The model under review builds one solid part; all positions refer to its coordinate system, in mm. Round coordinates to 2 decimals unless told otherwise and drop trailing zeros. Write each loop counter-clockwise with the first axis right and the second up, starting at its lowest first coordinate (ties: lowest second). Pieces come first, ordered by that corner, then holes. Notation, with made-up numbers: M 16.25,26.25 L 52.25,26.25 A36 ccw 52.25,65.25 Z; hole C 53.25,88.25 d1. An arc over 180 degrees is marked long. Write item = value, one per line. Start each with the question number.
Item 1: Take a section at A-A, the plane z = 45.4. Give the boundary of the cut face in (x, y).
Item 2: The part is to be moulded in two halves that separate along Z. For faces 1 (the flat face through (-1, 0, 24)), 2 (the cylindrical face through (8.689, 14.506, 36.984)), 3 (the cylindrical face through (8.69, 14.51, -31.26)), say which applies: +Z half, -Z half, draft (parallel to the pull), parting line (faces both ways), or undercut.
Item 3: For pin 1 Ø12 at (y, z) = (21, 13.5) entering from -X; pin 2 Ø1 at (x, y) = (-3.5, 17.5) entering from +Z; pin 3 Ø6 at (x, y) = (17.5, 30) entering from +Z, all flat-tipped, find the tip position at first contact; note any pin that passes through.
Item 4: Take a section at B-B, the plane y = 33. Give the number of separate pieces and of enclosed holes in the cut face, plus the area to 3 significant figures.
Item 5: To check wall thickness, follow line 1 along Z through (x, y) = (-0.5, 21); line 2 along X through (y, z) = (19.5, 28); line 3 along X through (y, z) = (15.5, 21.5). State the ranges of each line that lie inside material, in increasing order.
from build123d import *

# Parameters (mm, degrees)
SKETCH1_R                 = 50.8
SKETCH1_R_2               = 23.5
BOSS_EXTRUDE1_DEPTH       = 7.7
SKETCH3_R                 = 50.8
SKETCH3_R_2               = 30
BOSS_EXTRUDE2_DEPTH       = 9.7625
SKETCH4_R                 = 50.8
SKETCH4_R_2               = 40
BOSS_EXTRUDE3_DEPTH       = 19.05
SKETCH5_R                 = 3
CUT_EXTRUDE1_DEPTH        = 4.7625
CHAMFER1_SIZE             = 1.2
CUT_EXTRUDE4_DEPTH        = 81.58810493
M4X0_7_TAPPED_HOLE1_D     = 3.3
M4X0_7_TAPPED_HOLE1_DEPTH = 36.5135


with BuildPart() as part:
    # Sketch1 → Boss-Extrude1 (new body)
    with BuildSketch(Plane(origin=(0, 0, 0), x_dir=(1, 0, 0), z_dir=(0, 1, 0))):
        with Locations(Location((0, 0, 0), (0, 0, 90))):
            Circle(SKETCH1_R)
        with Locations(Location((0, 0, 0), (0, 0, 90))):
            Circle(SKETCH1_R_2, mode=Mode.SUBTRACT)
    extrude(amount=BOSS_EXTRUDE1_DEPTH)

    # Sketch3 → Boss-Extrude2 (add)
    with BuildSketch(Plane(origin=(0, 7.7, 0), x_dir=(1, 0, 0), z_dir=(0, 1, 0))):
        with Locations(Location((0, 0, 0), (0, 0, 90))):
            Circle(SKETCH3_R)
        with Locations(Location((0, 0, 0), (0, 0, 270))):
            Circle(SKETCH3_R_2, mode=Mode.SUBTRACT)
    extrude(amount=BOSS_EXTRUDE2_DEPTH)

    # Sketch4 → Boss-Extrude3 (add)
    with BuildSketch(Plane(origin=(0, 17.4625, 0), x_dir=(1, 0, 0), z_dir=(0, 1, 0))):
        with Locations(Location((0, 0, 0), (0, 0, 90))):
            Circle(SKETCH4_R)
        with Locations(Location((0, 0, 0), (0, 0, 90))):
            Circle(SKETCH4_R_2, mode=Mode.SUBTRACT)
    extrude(amount=BOSS_EXTRUDE3_DEPTH)

    # Sketch5 → Cut-Extrude1 (cut)
    with BuildSketch(Plane(origin=(0, 17.4625, 0), x_dir=(1, 0, 0), z_dir=(0, 1, 0))):
        with BuildLine():
            ThreePointArc((-38, 0), (-35, -3), (-32, 0))
            Line((-32, 0), (-38, 0))
        make_face()
        with BuildLine():
            Line((-38, 0), (-32, 0))
            ThreePointArc((-32, 0), (-35, 3), (-38, 0))
        make_face()
        with Locations(Location((-33.445048203, 10.316431104, 0), (0, 0, 270))):
            Circle(SKETCH5_R)
        with Locations(Location((-28.918357101, 19.716202032, 0), (0, 0, 270))):
            Circle(SKETCH5_R)
        with Locations(Location((-21.822143065, 27.364101886, 0), (0, 0, 270))):
            Circle(SKETCH5_R)
        with Locations(Location((-12.786935853, 32.580581203, 0), (0, 0, 270))):
            Circle(SKETCH5_R)
        with Locations(Location((-2.615553276, 34.902132901, 0), (0, 0, 270))):
            Circle(SKETCH5_R)
        with Locations(Location((7.788232688, 34.122476926, 0), (0, 0, 270))):
            Circle(SKETCH5_R)
        with Locations(Location((17.5, 30.310889132, 0), (0, 0, 270))):
            Circle(SKETCH5_R)
        with Locations(Location((25.656815514, 23.806045822, 0), (0, 0, 270))):
            Circle(SKETCH5_R)
        with Locations(Location((31.533910377, 15.185930869, 0), (0, 0, 270))):
            Circle(SKETCH5_R)
        with Locations(Location((34.609078918, 5.216479316, 0), (0, 0, 270))):
            Circle(SKETCH5_R)
        with Locations(Location((34.609078918, -5.216479316, 0), (0, 0, 270))):
            Circle(SKETCH5_R)
        with Locations(Location((31.533910377, -15.185930869, 0), (0, 0, 270))):
            Circle(SKETCH5_R)
        with Locations(Location((17.5, -30.310889132, 0), (0, 0, 270))):
            Circle(SKETCH5_R)
        with Locations(Location((7.788232688, -34.122476926, 0), (0, 0, 270))):
            Circle(SKETCH5_R)
        with Locations(Location((-2.615553276, -34.902132901, 0), (0, 0, 270))):
            Circle(SKETCH5_R)
        with Locations(Location((-12.786935853, -32.580581203, 0), (0, 0, 270))):
            Circle(SKETCH5_R)
        with Locations(Location((-21.822143065, -27.364101886, 0), (0, 0, 270))):
            Circle(SKETCH5_R)
        with Locations(Location((-28.918357101, -19.716202032, 0), (0, 0, 270))):
            Circle(SKETCH5_R)
        with Locations(Location((-33.445048203, -10.316431104, 0), (0, 0, 270))):
            Circle(SKETCH5_R)
        with Locations(Location((25.656815514, -23.806045822, 0), (0, 0, 270))):
            Circle(SKETCH5_R)
    extrude(amount=-CUT_EXTRUDE1_DEPTH, mode=Mode.SUBTRACT)

    # Chamfer1
    chamfer1_edges = [part.edges().sort_by_distance(p)[0] for p in [
        (-12.786935853, 17.4625, 29.580581203),
        (-2.615553276, 17.4625, 31.902132901),
        (7.788232688, 17.4625, 31.122476926),
        (17.5, 17.4625, 27.310889132),
        (31.533910377, 17.4625, 12.185930869),
        (34.609078918, 17.4625, 2.216479316),
        (34.609078918, 17.4625, -8.216479316),
        (31.533910377, 17.4625, -18.185930869),
        (25.656815514, 17.4625, -26.806045822),
        (17.5, 17.4625, -33.310889132),
        (7.788232688, 17.4625, -37.122476926),
        (-2.615553276, 17.4625, -37.902132901),
        (-12.786935853, 17.4625, -35.580581203),
        (-21.822143065, 17.4625, -30.364101886),
        (-28.918357101, 17.4625, -22.716202032),
        (-33.445048203, 17.4625, -13.316431104),
        (25.656815514, 17.4625, 20.806045822),
        (-33.445048203, 17.4625, 7.316431104),
        (-28.918357101, 17.4625, 16.716202032),
        (-21.822143065, 17.4625, 24.364101886),
        (-38, 17.4625, 0),
    ]]
    chamfer(chamfer1_edges, length=CHAMFER1_SIZE)

    # Sketch9 → Cut-Extrude4 (cut, through all)
    with BuildSketch(Plane(origin=(0, 36.5125, 0), x_dir=(1, 0, 0), z_dir=(0, 1, 0))):
        with BuildLine():
            Line((-16.632498309, 48), (0, 48))
            Line((0, 48), (16.632498309, 48))
            ThreePointArc((16.632498309, 48), (0, 50.8), (-16.632498309, 48))
        make_face()
    extrude(amount=-CUT_EXTRUDE4_DEPTH, mode=Mode.SUBTRACT)

    # M4x0.7 Tapped Hole1
    with Locations(Plane(origin=(0, 36.5125, 0), x_dir=(1, 0, 0), z_dir=(0, 1, 0))):
        with Locations((0, -45.4), (0, 0), (-44.261727213, 10.102450402), (-35.495149304, -28.306437004), (-19.698321756, 40.903986603), (19.698321756, 40.903986603), (44.261727213, 10.102450402), (35.495149304, -28.306437004)):
            Hole(M4X0_7_TAPPED_HOLE1_D / 2, depth=M4X0_7_TAPPED_HOLE1_DEPTH)


solid = part.part
Response values:
q1.outline = M -22.79,0 L -1.65,0 L -1.65,36.51 L -22.79,36.51 Z; M 1.65,0 L 22.79,0 L 22.79,36.51 L 1.65,36.51 Z
q2.face_1 = draft
q2.face_2 = undercut
q2.face_3 = undercut
q3.pin_1 = -50.24
q3.pin_2 = 50.71
q3.pin_3 = 48.69
q4.separate_pieces = 1
q4.enclosed_holes = 8
q4.area = 2,960 mm2
q5.line_1 = -48 to -40, 40 to 43.83, 46.97 to 50.8
q5.line_2 = -42.39 to -37.12, -33.87 to -28.57, 28.57 to 33.87, 37.12 to 42.39
q5.line_3 = -46.03 to -31.33, -26.51 to -20.92, 20.92 to 23.74, 27.58 to 46.03
